```python
from build123d import *

# Parameters (mm, degrees)
F1_W     = 6.5
F1_H     = 21
F1_R     = 7.5
F2_DEPTH = 3
F4_DEPTH = 3


# Not quite as in the source:
# - a feature names something its author has since deleted; it is built from what else it names


with BuildPart() as f2:
    # F1 (on Front) → F2 (new body)
    with BuildSketch(Plane.XZ):
        Polygon((33, 5), (33, 19), (-33, 19), (-33, 5), (-36, 5), (-36, -5), (-33, -5), (-33, -19), (-28, -19), (-28, -22), (-18, -22), (-18, -19), (0, -19), (18, -19), (18, -22), (28, -22), (28, -19), (33, -19), (33, -5), (36, -5), (36, 5), align=None)
        with Locations((-26.75, -5.25)):
            Rectangle(F1_W, F1_H, mode=Mode.SUBTRACT)
        Circle(F1_R, mode=Mode.SUBTRACT)
    extrude(amount=F2_DEPTH)

    # F3 (on face) → F4 (cut, through all)
    with BuildSketch(Plane.XZ.offset(3)):
        Polygon((10.5, -16), (10.5, -19), (13.5, -19), (13.5, -16), (15, -16), (15, -13.5), (13.5, -13.5), (13.5, -11.5), (10.5, -11.5), (10.5, -13.5), (9, -13.5), (9, -16), align=None)
        Polygon((-13.5, -19), (-10.5, -19), (-10.5, -16), (-9, -16), (-9, -13.5), (-10.5, -13.5), (-10.5, -11.5), (-13.5, -11.5), (-13.5, -13.5), (-15, -13.5), (-15, -16), (-13.5, -16), align=None)
        Polygon((30, 9.5), (33, 9.5), (33, 12.5), (30, 12.5), (30, 14), (27.5, 14), (27.5, 12.5), (25.5, 12.5), (25.5, 9.5), (27.5, 9.5), (27.5, 8), (30, 8), align=None)
        Polygon((-33, 12.5), (-33, 9.5), (-30, 9.5), (-30, 8), (-27.5, 8), (-27.5, 9.5), (-25.5, 9.5), (-25.5, 12.5), (-27.5, 12.5), (-27.5, 14), (-30, 14), (-30, 12.5), align=None)
    extrude(amount=-F4_DEPTH, mode=Mode.SUBTRACT)


solid = f2.part
```
The listing builds one solid part. Answer for the finished solid, in the listing's coordinates (mm). A direction names the side the tool comes from. Give positions to 0.01 mm unless a question says otherwise; leave off trailing zeros. Order: outer loops, then holes, each group sorted by start corner. A loop starts at its lowest first (then second) coordinate and runs counter-clockwise, first axis right, second up. Notation, with made-up numbers: (66, 53) -> (122, 53) arc R36 ccw to (122, 89) -> close; hole circle Ø7 at (22, 51.25). An arc over 180 degrees is marked (long way). Answer as a JSON object with one key per item and string values. Group by question number.
Item 1: A tool of negligible diameter and unlimited length cuts with its end or side. For faces 4 (the flat face through (-28, -1, -20)), 5 (the flat face through (33, -1, -12)), 6 (the flat face through (-34, -1, 5)), 7 (the flat face through (-29, -2, 8)), 8 (the flat face through (33, -1, 16)), from which of +Z, -Z, +X, -X, +Y, -Y can it reach the whole face along a straight path? Write none if from no direction.
Item 2: The part is cut by section A-A on z = 6. Write down the section's boundary in (x, y), and give its area (3 significant figures).
Item 3: The part is cut by section C-C on z = -14.5. Write down the section's boundary in (x, y).
Item 4: Determine the mould class of faces 1 (the flat face through (-10.5, -2, -13)), 2 (the flat face through (0, -1, -19)), 3 (the flat face through (-25.5, -2, 11)) for opening direction Z: pulls with the +Z half, pulls with the -Z half, needs draft (parallel to the pull), parting line crosses it, or undercut.
Item 5: Consider L1, parallel to X at y = -2.55, z = -15.5; L2, parallel to X at y = -1.6, z = -9.5; L3, parallel to Z at x = 0, y = -0.7. Determine where each line is inside the solid, lowest interval first. Write a range as from..to.
Item 6: The part is cut by section B-B on x = 0. Write down the section's boundary in (y, z), and give its area (3 significant figures).
Item 7: Flat-ended cylindrical pins translate along their axes: pin 1 (0.9 mm diameter, centred on y = -1, z = -17.5, fed in from +X); pin 2 (1.5 mm diameter, centred on y = -1.5, z = 11.5, fed in from -X). Find the tip coordinate at first contact, or state that the pin passes through.
Item 8: The part is cut by section D-D on z = 0. Write down the section's boundary in (x, y).
Result set:
{
 "1": {"face 4": "-Z, -X, +Y, -Y", "face 5": "-Z, +X, +Y, -Y", "face 6": "+Z, -X, +Y, -Y", "face 7": "+Y, -Y", "face 8": "+Z, +X, +Y, -Y"},
 "2": {"outline": "(-33, -3) -> (-4.5, -3) -> (-4.5, 0) -> (-33, 0) -> close; (4.5, -3) -> (33, -3) -> (33, 0) -> (4.5, 0) -> close", "area": "171 mm²"},
 "3": {"outline": "(-33, -3) -> (-30, -3) -> (-30, 0) -> (-33, 0) -> close; (-23.5, -3) -> (-15, -3) -> (-15, 0) -> (-23.5, 0) -> close; (-9, -3) -> (9, -3) -> (9, 0) -> (-9, 0) -> close; (15, -3) -> (33, -3) -> (33, 0) -> (15, 0) -> close"},
 "4": {"face 1": "needs draft", "face 2": "pulls with the -Z half", "face 3": "undercut"},
 "5": {"L1": "-33..-30, -23.5..-15, -9..9, 15..33", "L2": "-33..-30, -23.5..33", "L3": "-19..-7.5, 7.5..19"},
 "6": {"outline": "(-3, -19) -> (0, -19) -> (0, -7.5) -> (-3, -7.5) -> close; (-3, 7.5) -> (0, 7.5) -> (0, 19) -> (-3, 19) -> close", "area": "69.0 mm²"},
 "7": {"pin 1": "x = 33", "pin 2": "x = -25.5"},
 "8": {"outline": "(-36, -3) -> (-30, -3) -> (-30, 0) -> (-36, 0) -> close; (-23.5, -3) -> (-7.5, -3) -> (-7.5, 0) -> (-23.5, 0) -> close; (7.5, -3) -> (36, -3) -> (36, 0) -> (7.5, 0) -> close"}
}
